```python
from build123d import *

# Parameters (mm, degrees)
F1_DEPTH = 80
F2_R     = 3.25
F3_DEPTH = 20.001
F4_R     = 6
F4_R_2   = 3.25
F5_DEPTH = 6


with BuildPart() as f1:
    # F0 (on Front) → F1 (new body)
    with BuildSketch(Plane.XZ):
        Polygon((-14, 0), (0, 0), (0, 20), (-23, 20), (-23, 8.5), (-14, 8.5), align=None)
    extrude(amount=F1_DEPTH)

    # F2 (on face) → F3 (cut, through all)
    with BuildSketch(Plane.XY.offset(20)):
        with Locations((-7.5, -15)):
            Circle(F2_R)
        with Locations((-7.5, -65)):
            Circle(F2_R)
    extrude(amount=-F3_DEPTH, mode=Mode.SUBTRACT)

    # F4 (on face) → F5 (cut)
    with BuildSketch(Plane.XY.offset(20)):
        with Locations((-7.5, -15)):
            Circle(F4_R)
        with Locations((-7.5, -15)):
            Circle(F4_R_2, mode=Mode.SUBTRACT)
        with Locations((-7.5, -65)):
            Circle(F4_R)
        with Locations((-7.5, -65)):
            Circle(F4_R_2, mode=Mode.SUBTRACT)
    extrude(amount=-F5_DEPTH, mode=Mode.SUBTRACT)


solid = f1.part
```
The model under review builds one solid part; all positions refer to its coordinate system, in mm. A direction names the side the tool comes from. Round coordinates to 2 decimals unless told otherwise and drop trailing zeros. Loops run counter-clockwise (first coordinate to the right, second up) from the corner with the lowest first, then second, coordinate; pieces in that order, holes last.
Item 1: Mouldability with a two-part tool opening along Y and no side actions: class faces 1 (the face through (-9, -80, 12)), 2 (the face through (-9.895, -12.803, 7.098)), 3 (the face through (0, -39, 10)) as released by +Y, released by -Y, zero draft, split by the parting line, or undercut.
Determined:
face 1: released by -Y
face 2: undercut
face 3: zero draft
Item 2: For faces 4 (the face through (-7.923, -61.778, 7.098)), 5 (the face through (-5, -68, 14)), 6 (the face through (-14, -39, 4)), list the 3-axis set-ups (+Z, -Z, +X, -X, +Y, -Y) from which the entire face can be reached by the end or side of a thin tool; tool diameter is ignored.
Determined:
face 4: +Z, -Z
face 5: +Z
face 6: -Z, -X, +Y, -Y
Item 3: Take a section at A-A (x = -7.5). Write out the cut boundary in (y, z), then the cut area to 3 significant figures.
Determined:
outline: (-80, 0) - (-68.25, 0) - (-68.25, 14) - (-71, 14) - (-71, 20) - (-80, 20) - close; (-61.75, 0) - (-18.25, 0) - (-18.25, 14) - (-21, 14) - (-21, 20) - (-59, 20) - (-59, 14) - (-61.75, 14) - close; (-11.75, 0) - (0, 0) - (0, 20) - (-9, 20) - (-9, 14) - (-11.75, 14) - close
area: 1,270 mm2
Item 4: Take a section at B-B (y = -15). Write out the cut boundary in (x, z).
Determined:
outline: (-23, 8.5) - (-14, 8.5) - (-14, 0) - (-10.75, 0) - (-10.75, 14) - (-13.5, 14) - (-13.5, 20) - (-23, 20) - close; (-4.25, 0) - (0, 0) - (0, 20) - (-1.5, 20) - (-1.5, 14) - (-4.25, 14) - close
Item 5: Take a section at C-C (z = 4). Write out the cut boundary in (x, y), then the cut area to 3 significant figures.
Determined:
outline: (-14, -80) - (0, -80) - (0, 0) - (-14, 0) - close; hole circle Ø6.5 at (-7.5, -65); hole circle Ø6.5 at (-7.5, -15)
area: 1,050 mm2
Item 6: For line 1 (Y direction, x = -7.5, z = 16); line 2 (Y direction, x = -7.5, z = 8.5); line 3 (X direction, y = -32.5, z = 2), list the stretches that pass through material, from the lowest coordinate up.
Determined:
line 1: y = -80 to -71, -59 to -21, -9 to 0
line 2: y = -80 to -68.25, -61.75 to -18.25, -11.75 to 0
line 3: x = -14 to 0
Item 7: Take a section at D-D (y = -34). Write out the cut boundary in (x, z), then the cut area to 4 significant figures.
Determined:
outline: (-23, 8.5) - (-14, 8.5) - (-14, 0) - (0, 0) - (0, 20) - (-23, 20) - close
area: 383.5 mm2
Item 8: Clearance check with flat-ended pins moving along their axes: pin 1 Ø2.5 at (x, y) = (-20, -39.5) entering from -Z; pin 2 Ø4 at (y, z) = (-21.5, 3) entering from -X; pin 3 Ø11 at (x, y) = (-7.5, -15) entering from +Z. State where each tip first meets the part, or that it passes through.
Determined:
pin 1: stops at z = 8.5
pin 2: stops at x = -14
pin 3: stops at z = 14
